Study the drawing (mm; zero at the part's minimum x, y, z) and answer. A direction names the side the tool comes from. Round coordinates to 2 decimals unless told otherwise and drop trailing zeros. Loops run counter-clockwise (first coordinate to the right, second up) from the corner with the lowest first, then second, coordinate; pieces in that order, holes last. Notation, with made-up numbers: (78.5, 80.25) -> (119.5, 80.25) arc R17 ccw to (119.5, 105.25) -> close; hole circle Ø10 at (72, 67). An arc over 180 degrees is marked (long way). Write each question's results on one line, items separated by ' | '. Start each with the question number.
(1) For the marked faces 1 and 2, determine the directions among +Z, -Z, +X, -X, +Y, -Y from which every point of the face is accessible in a straight line to the end or side of a thin tool.
(2) Determine the mould class of the marked faces 3, 4, 5 and 6 for opening direction Y: released by +Y, released by -Y, zero draft, split by the parting line, or undercut.
(3) The part is cut by section B-B (x = 9.25). Determine the outline of the cut face in (y, z).
(4) A flat-ended cylindrical pin translates along its axis: pin 1 (3 mm diameter, centred on x = 5.5, y = 25.5, fed in from -Z). Find the tip coordinate at first contact, or state that the pin passes through.
(5) The part is cut by section C-C (y = 16). Determine the outline of the cut face in (x, z), plus the area to 3 significant figures.
(6) The part is cut by section A-A (z = 3.5). Determine the outline of the cut face in (x, y), plus the area to 3 significant figures.
(7) Straight lines are drawn through the part: probe 1 along Y at (x, z) = (1, 4.25); probe 2 along Z at (x, y) = (3.25, 28). For each, find the intervals that lie inside material, in ascending order.
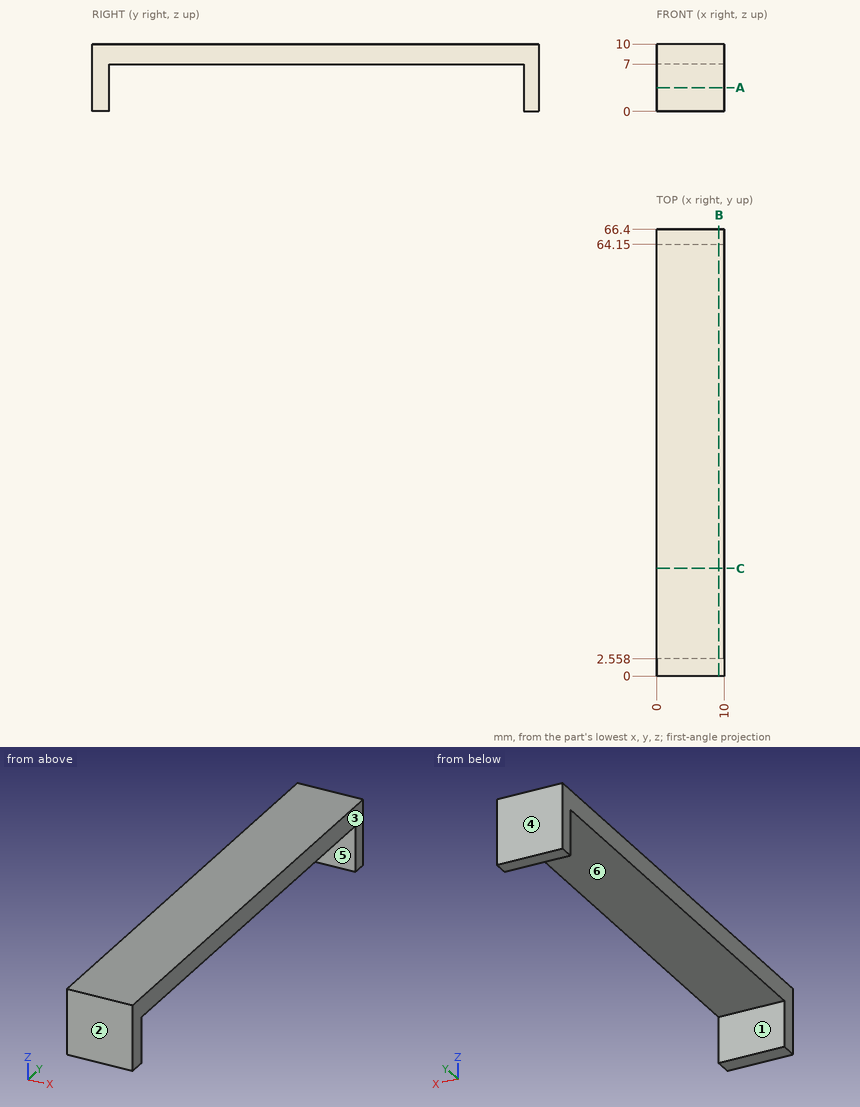
Checked values:
1) face 1: -Z, +X, -X | face 2: +Z, -Z, +X, -X, -Y
2) face 3: zero draft | face 4: released by +Y | face 5: undercut | face 6: undercut
3) outline: (0, 0) -> (2.56, 0) -> (2.56, 7) -> (64.15, 7) -> (64.15, 0) -> (66.4, 0) -> (66.4, 10) -> (0, 10) -> close
4) pin 1: stops at z = 7
5) outline: (0, 7) -> (10, 7) -> (10, 10) -> (0, 10) -> close | area: 30.0 mm2
6) outline: (0, 0) -> (10, 0) -> (10, 2.56) -> (0, 2.56) -> close; (0, 64.15) -> (10, 64.15) -> (10, 66.4) -> (0, 66.4) -> close | area: 48.1 mm2
7) probe 1: y = 0 to 2.56, 64.15 to 66.4 | probe 2: z = 7 to 10
